from build123d import *

# Parameters (mm, degrees)
SKETCH1_W              = 177.8
SKETCH1_H              = 39.878
BOSS_EXTRUDE1_DEPTH    = 11.049
F_10_32_TAPPED_HOLE1_D = 4.0386
BOSS_EXTRUDE2_DEPTH    = 2.032


with BuildPart() as part:
    # Sketch1 → Boss-Extrude1 (new body)
    with BuildSketch(Plane(origin=(0, 0, 0), x_dir=(0, 0, -1), z_dir=(1, 0, 0))):
        Rectangle(SKETCH1_W, SKETCH1_H)
        with BuildLine():
            Line((-73.9252522, 6.6675), (73.9252522, 6.6675))
            ThreePointArc((73.9252522, 6.6675), (80.5927522, 0), (73.9252522, -6.6675))
            Line((73.9252522, -6.6675), (-73.9252522, -6.6675))
            ThreePointArc((-73.9252522, -6.6675), (-80.5927522, 0), (-73.9252522, 6.6675))
        make_face(mode=Mode.SUBTRACT)
    extrude(amount=BOSS_EXTRUDE1_DEPTH)

    # #10-32 Tapped Hole1 (through all)
    with Locations(Plane(origin=(11.049, 0, 0), x_dir=(0, 0, -1), z_dir=(1, 0, 0))):
        with Locations((-82.55, 13.589), (-82.55, -13.589), (0, -13.589), (82.55, -13.589), (82.55, 13.589), (0, 13.589)):
            Hole(F_10_32_TAPPED_HOLE1_D / 2)

    # Sketch5 → Boss-Extrude2 (add)
    with BuildSketch(Plane.ZY):
        with BuildLine():
            Line((35.243819624, 6.6675), (35.243819624, 6.6421))
            ThreePointArc((35.243819624, 6.6421), (29.1577522, 0), (35.243819624, -6.6421))
            Line((35.243819624, -6.6421), (35.243819624, -6.6675))
            Line((35.243819624, -6.6675), (-73.9252522, -6.6675))
            ThreePointArc((-73.9252522, -6.6675), (-80.5927522, 0), (-73.9252522, 6.6675))
            Line((-73.9252522, 6.6675), (35.243819624, 6.6675))
        make_face()
    extrude(amount=-BOSS_EXTRUDE2_DEPTH)


solid = part.part
Geometry: final body of the model. Coordinates: model frame, mm. A direction names the side the tool comes from. Give positions to 0.01 mm unless a question says otherwise; leave off trailing zeros. Order: outer loops, then holes, each group sorted by start corner. A loop starts at its lowest first (then second) coordinate and runs counter-clockwise, first axis right, second up. Notation, with made-up numbers: (73, 74) -> (112, 74) arc R24 cw to (112, 105) -> close; hole circle Ø11 at (75.5, -19). An arc over 180 degrees is marked (long way). Answer as a JSON object with one key per item and string values.
Q1. Section C-C (z = -82.55). Output: boundary loops of the cut face in (x, y).
Entries:
{"outline": "(0, -19.94) -> (11.05, -19.94) -> (11.05, -15.61) -> (0, -15.61) -> close; (0, -11.57) -> (11.05, -11.57) -> (11.05, 11.57) -> (0, 11.57) -> close; (0, 15.61) -> (11.05, 15.61) -> (11.05, 19.94) -> (0, 19.94) -> close"}
Q2. Section B-B (y = 0). Output: boundary loops of the cut face in (x, z).
Entries:
{"outline": "(0, -88.9) -> (11.05, -88.9) -> (11.05, -80.59) -> (2.03, -80.59) -> (2.03, 29.16) -> (0, 29.16) -> close; (0, 80.59) -> (11.05, 80.59) -> (11.05, 88.9) -> (0, 88.9) -> close"}
Q3. Material intervals for probe 1 along Y at (x, z) = (3, 82.55); probe 2 along Y at (x, z) = (2.75, 0); probe 3 along Y at (x, z) = (3.5, -11), sorted ascending.
Entries:
{"probe 1": "y = -19.94 to -15.61, -11.57 to 11.57, 15.61 to 19.94", "probe 2": "y = -19.94 to -15.61, -11.57 to -6.67, 6.67 to 11.57, 15.61 to 19.94", "probe 3": "y = -19.94 to -6.67, 6.67 to 19.94"}
Q4. Section D-D (x = 3.5). State how many separate pieces and enclosed holes the cut face has, plus the area to 3 significant figures.
Entries:
{"separate pieces": "1", "enclosed holes": "7", "area": "4,900 mm^2"}
Q5. Draft query along Z for faces 1 (the flat face through (5, 0, -88.9)), 2 (the cylindrical face through (5.447, -11.587, -0.263)), 3 (the flat face through (5, -19.939, 1)). Return one class per face: released by +Z, released by -Z, zero draft, split by the parting line, or undercut.
Entries:
{"face 1": "released by -Z", "face 2": "undercut", "face 3": "zero draft"}
Q6. Access query for faces 4 (the cylindrical face through (5.45, -0.15, 80.59)), 5 (the flat face through (2.032, 0, -22)), 6 (the flat face through (11.049, 9, 1)). Directions: +Z, -Z, +X, -X, +Y, -Y. A direction counts if a zero-diameter tool reaches every point of the face in a straight line with its end or side. Return the directions, or none.
Entries:
{"face 4": "+X, -X", "face 5": "+X", "face 6": "+Z, -Z, +X, +Y, -Y"}
Q7. Section A-A (z = 49). Output: boundary loops of the cut face in (x, y), plus the area to 3 significant figures.
Entries:
{"outline": "(0, -19.94) -> (11.05, -19.94) -> (11.05, -6.67) -> (0, -6.67) -> close; (0, 6.67) -> (11.05, 6.67) -> (11.05, 19.94) -> (0, 19.94) -> close", "area": "293 mm^2"}
Q8. First-contact query: pin 1 (3.5 mm diameter, centred on y = -13.589, z = 0, fed in from +X); pin 2 (6.5 mm diameter, centred on y = 0.5, z = -30, fed in from +X). Flat tips, straight axial feed; report the tip coordinate or a pass-through.
Entries:
{"pin 1": "passes through", "pin 2": "stops at x = 2.03"}
